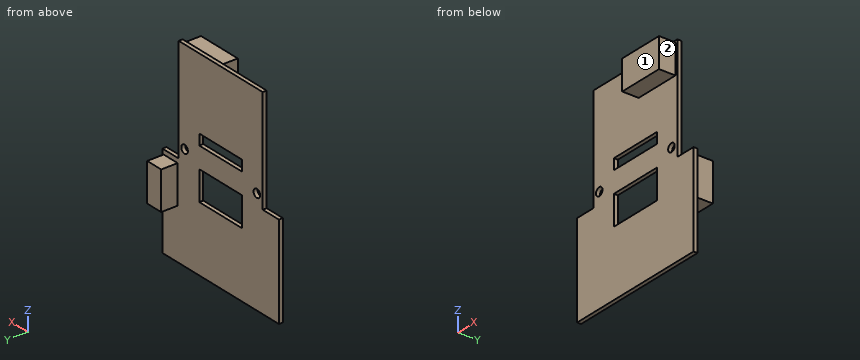
```python
from build123d import *

# Parameters (mm, degrees)
SKETCH_1_R      = 1.25
SKETCH_1_W      = 16.323541982
SKETCH_1_H      = 8.961255986
SKETCH_1_H_2    = 3.269836796
EXTRUDE_1_DEPTH = 1.2
SKETCH_2_W      = 5.33414326
SKETCH_2_H      = 11.592185383
EXTRUDE_2_DEPTH = 5
SKETCH_3_W      = 14
SKETCH_3_H      = 9
EXTRUDE_3_DEPTH = 5


with BuildPart() as part:
    # 草图1 → 凸台-拉伸1 (new body)
    with BuildSketch(Plane(origin=(0, 0, 0), x_dir=(1, 0, 0), z_dir=(0, 1, 0))):
        Polygon((16, 0), (16, -32), (-16, -32), (-16, 0), (-22.15, 0), (-22.15, 28.4), (22.15, 28.4), (22.15, 0), align=None)
        with Locations(Location((13.75, -3.5, 0), (0, 0, 270))):
            Circle(SKETCH_1_R, mode=Mode.SUBTRACT)
        with Locations(Location((-13.75, -3.5, 0), (0, 0, 90))):
            Circle(SKETCH_1_R, mode=Mode.SUBTRACT)
        with Locations((0, 3.973903908)):
            Rectangle(SKETCH_1_W, SKETCH_1_H, mode=Mode.SUBTRACT)
        with Locations((0, -8.562744205)):
            Rectangle(SKETCH_1_W, SKETCH_1_H_2, mode=Mode.SUBTRACT)
    extrude(amount=EXTRUDE_1_DEPTH)

    # 草图2 → 凸台-拉伸2 (add)
    with BuildSketch(Plane(origin=(0, 1.2, 0), x_dir=(1, 0, 0), z_dir=(0, 1, 0))):
        with Locations((19.068534732, 7.22523066)):
            Rectangle(SKETCH_2_W, SKETCH_2_H)
    extrude(amount=EXTRUDE_2_DEPTH)

    # 草图3 → 凸台-拉伸3 (add)
    with BuildSketch(Plane.XZ):
        with Locations((8.26747858, 26.972724501)):
            Rectangle(SKETCH_3_W, SKETCH_3_H)
    extrude(amount=EXTRUDE_3_DEPTH)


solid = part.part
```
Design review of the part built by this model. Coordinates are the model's own, in mm. Face numbers are marked on the shaded views. Give positions to 0.01 mm unless a question says otherwise; leave off trailing zeros. Order: outer loops, then holes, each group sorted by start corner. A loop starts at its lowest first (then second) coordinate and runs counter-clockwise, first axis right, second up. Notation, with made-up numbers: (58, 55) -> (70, 55) arc R27 ccw to (70, 92) -> close; hole circle Ø3 at (-36.75, 85). An arc over 180 degrees is marked (long way). Write each question's results on one line, items separated by ' | '. Start each with the question number.
Q1. Add section A-A on z = 3.5. Give the boundary of the cut face in (x, y), and give its area (3 significant figures).
Q2. For pin 1 (2.5 mm diameter, centred on x = 19.5, y = 3.5, fed in from +Z); pin 2 (1.3 mm diameter, centred on x = -19.5, y = 1, fed in from +Z); pin 3 (4 mm diameter, centred on y = 4.5, z = -9, fed in from +X), all flat-tipped, find the tip position at first contact; note any pin that passes through.
Q3. Mouldability with a two-part tool opening along Y and no side actions: class the marked faces 1 and 2 as +Y half, -Y half, draft (parallel to the pull), parting line (faces both ways), or undercut.
Q4. Add section D-D on z = -5. Give the boundary of the cut face in (x, y), and give its area (3 significant figures).
Q5. Wall thickness on L1, parallel to X at y = 0.75, z = 3.5; L2, parallel to Z at x = -13.75, y = 0.8; L3, parallel to Y at x = 2.5, z = -21: over which ranges is each line inside the solid? List them lowest first. Write a range as from..to.
Q6. Add section C-C on x = -2. Give the boundary of the cut face in (y, z).
Q7. Add section B-B on x = 13.75. Give the boundary of the cut face in (y, z).
Found:
1) outline: (-16, 0) -> (-15, 0) -> (-15, 1.2) -> (-16, 1.2) -> close; (-12.5, 0) -> (12.5, 0) -> (12.5, 1.2) -> (-12.5, 1.2) -> close; (15, 0) -> (16, 0) -> (16, 1.2) -> (15, 1.2) -> close | area: 32.4 mm2
2) pin 1: stops at z = -1.43 | pin 2: stops at z = 0 | pin 3: stops at x = 21.74
3) face 1: -Y half | face 2: draft
4) outline: (-22.15, 0) -> (-8.16, 0) -> (-8.16, 1.2) -> (-22.15, 1.2) -> close; (8.16, 0) -> (22.15, 0) -> (22.15, 1.2) -> (21.74, 1.2) -> (21.74, 6.2) -> (16.4, 6.2) -> (16.4, 1.2) -> (8.16, 1.2) -> close | area: 60.2 mm2
5) L1: x = -16..-15, -12.5..12.5, 15..16 | L2: z = -28.4..2.25, 4.75..32 | L3: y = 0..1.2
6) outline: (0, -28.4) -> (1.2, -28.4) -> (1.2, -8.45) -> (0, -8.45) -> close; (0, 0.51) -> (1.2, 0.51) -> (1.2, 6.93) -> (0, 6.93) -> close; (0, 10.2) -> (1.2, 10.2) -> (1.2, 32) -> (0, 32) -> close
7) outline: (-5, 22.47) -> (0, 22.47) -> (0, 4.75) -> (1.2, 4.75) -> (1.2, 32) -> (0, 32) -> (0, 31.47) -> (-5, 31.47) -> close; (0, -28.4) -> (1.2, -28.4) -> (1.2, 2.25) -> (0, 2.25) -> close
